Here's how the part is built. I have some questions about the finished solid (model axes, mm). A direction names the side the tool comes from. Coordinates: 2 decimals unless noted, no trailing zeros. Write each loop counter-clockwise with the first axis right and the second up, starting at its lowest first coordinate (ties: lowest second). Pieces come first, ordered by that corner, then holes. Notation, with made-up numbers: (18, -39.5) -> (41, -39.5) arc R27 ccw to (41, -15.5) -> close; hole circle Ø4 at (52, 20.25). An arc over 180 degrees is marked (long way). Answer in a Markdown table with one row per item. Add a question column.
from build123d import *

# Parameters (mm, degrees)
BOSS_EXTRUDE1_DEPTH = 15
SKETCH2_R           = 2.5
BOSS_EXTRUDE2_DEPTH = 2.5
FILLET1_R           = 1


with BuildPart() as part:
    # Sketch1 → Boss-Extrude1 (new, symmetric)
    with BuildSketch(Plane.XY):
        Polygon((-283.115153194, -200), (-283.115153194, 184.822832525), (-312.771891152, 214.573189293), (-282.723872007, 185), (282.728718813, 185), (312.776737958, 214.573189293), (283.12, 184.822832525), (283.12, -200), (313.12, -200), (313.12, 215), (-313.115153194, 215), (-313.115153194, -200), align=None)
    extrude(amount=BOSS_EXTRUDE1_DEPTH, both=True)

    # Sketch2 → Boss-Extrude2 (add, symmetric)
    with BuildSketch(Plane.ZY.offset(-283.12)):
        with BuildLine():
            Line((-15, -95.731232334), (-142.725217813, -153.297064452))
            ThreePointArc((-142.725217813, -153.297064452), (-144.870286213, -155.141843308), (-145.67073896, -157.855476088))
            Line((-145.67073896, -157.855476088), (-145.67073896, -195))
            ThreePointArc((-145.67073896, -195), (-144.206272866, -198.535533906), (-140.67073896, -200))
            Line((-140.67073896, -200), (140.67073896, -200))
            ThreePointArc((140.67073896, -200), (144.206272866, -198.535533906), (145.67073896, -195))
            Line((145.67073896, -195), (145.67073896, -157.855476088))
            ThreePointArc((145.67073896, -157.855476088), (144.870286213, -155.141843308), (142.725217813, -153.297064452))
            Line((142.725217813, -153.297064452), (15, -95.731232334))
            Line((15, -95.731232334), (-15, -95.731232334))
        make_face()
        with Locations(Location((-131.096268678, -157.855476088, 0), (0, 0, 270))):
            Circle(SKETCH2_R, mode=Mode.SUBTRACT)
        with Locations(Location((-131.096268678, -191.557763375, 0), (0, 0, 270))):
            Circle(SKETCH2_R, mode=Mode.SUBTRACT)
        with Locations(Location((131.096268678, -191.557763375, 0), (0, 0, 90))):
            Circle(SKETCH2_R, mode=Mode.SUBTRACT)
        with Locations(Location((131.096268678, -157.855476088, 0), (0, 0, 90))):
            Circle(SKETCH2_R, mode=Mode.SUBTRACT)
    boss_extrude2 = extrude(amount=BOSS_EXTRUDE2_DEPTH, both=True)

    # Mirror2: Boss-Extrude2 across plane
    add(boss_extrude2.mirror(Plane(origin=(0, 0, 0), x_dir=(0, 0, 1), z_dir=(1, 0, 0))))

    # Fillet1
    # the kernel refuses this fillet: 1 mm, written as the material it takes off along each edge
    with BuildSketch(Plane(origin=(-312.115153194, 214, -14), x_dir=(0, 0, -1), z_dir=(-1, 0, 0))) as fillet1_piece_1_section:
        Polygon((0, 0), (FILLET1_R * 1.02, 0), (FILLET1_R * 1.02, -FILLET1_R * 1.02), (0, -FILLET1_R * 1.02), align=None)
    fillet1_piece_1 = extrude(amount=FILLET1_R * 1.02, mode=Mode.PRIVATE)
    fillet1_piece_1 = fillet1_piece_1 - Plane(origin=(-312.115153194, 214, -14), x_dir=(0, -0.7071067811865475, 0.7071067811865475), z_dir=(-1, 0, 0)) * Sphere(FILLET1_R, mode=Mode.PRIVATE)
    add(fillet1_piece_1, mode=Mode.SUBTRACT)
    with BuildSketch(Plane(origin=(312.12, 214, -14), x_dir=(1, 0, 0), z_dir=(0, 1, 0))) as fillet1_piece_2_section:
        Polygon((0, 0), (FILLET1_R * 1.02, 0), (FILLET1_R * 1.02, FILLET1_R * 1.02), (0, FILLET1_R * 1.02), align=None)
    fillet1_piece_2 = extrude(amount=FILLET1_R * 1.02, mode=Mode.PRIVATE)
    fillet1_piece_2 = fillet1_piece_2 - Plane(origin=(312.12, 214, -14), x_dir=(-0.7071067811865475, 0, 0.7071067811865475), z_dir=(0, 1, 0)) * Sphere(FILLET1_R, mode=Mode.PRIVATE)
    add(fillet1_piece_2, mode=Mode.SUBTRACT)
    with BuildSketch(Plane(origin=(-312.115153194, 214, 14), x_dir=(0, 0, 1), z_dir=(-1, 0, 0))) as fillet1_piece_3_section:
        Polygon((0, 0), (FILLET1_R * 1.02, 0), (FILLET1_R * 1.02, FILLET1_R * 1.02), (0, FILLET1_R * 1.02), align=None)
    fillet1_piece_3 = extrude(amount=FILLET1_R * 1.02, mode=Mode.PRIVATE)
    fillet1_piece_3 = fillet1_piece_3 - Plane(origin=(-312.115153194, 214, 14), x_dir=(0, -0.7071067811865475, -0.7071067811865475), z_dir=(-1, 0, 0)) * Sphere(FILLET1_R, mode=Mode.PRIVATE)
    add(fillet1_piece_3, mode=Mode.SUBTRACT)
    with BuildSketch(Plane(origin=(312.12, 214, 14), x_dir=(1, 0, 0), z_dir=(0, 1, 0))) as fillet1_piece_4_section:
        Polygon((0, 0), (FILLET1_R * 1.02, 0), (FILLET1_R * 1.02, -FILLET1_R * 1.02), (0, -FILLET1_R * 1.02), align=None)
    fillet1_piece_4 = extrude(amount=FILLET1_R * 1.02, mode=Mode.PRIVATE)
    fillet1_piece_4 = fillet1_piece_4 - Plane(origin=(312.12, 214, 14), x_dir=(-0.7071067811865475, 0, -0.7071067811865475), z_dir=(0, 1, 0)) * Sphere(FILLET1_R, mode=Mode.PRIVATE)
    add(fillet1_piece_4, mode=Mode.SUBTRACT)
    with BuildSketch(Plane(origin=(-313.115153194, 214, -15), x_dir=(0, 0, 1), z_dir=(0, -1, 0)), Plane(origin=(313.12, -202.5, 15), x_dir=(-1, 0, 0), z_dir=(0, 1, 0))) as fillet1_piece_5:
        with BuildLine():
            CenterArc((FILLET1_R, -FILLET1_R), FILLET1_R, 90, 90)
            Line((0, -FILLET1_R), (0, 0))
            Line((0, 0), (FILLET1_R, 0))
        make_face()
    extrude(amount=416.5, mode=Mode.SUBTRACT)
    with BuildSketch(Plane(origin=(312.12, 215, -15), x_dir=(0, -1, 0), z_dir=(-1, 0, 0))) as fillet1_piece_6:
        with BuildLine():
            CenterArc((FILLET1_R, FILLET1_R), FILLET1_R, 180, 90)
            Line((0, FILLET1_R), (0, 0))
            Line((0, 0), (FILLET1_R, 0))
        make_face()
    extrude(amount=624.235153194, mode=Mode.SUBTRACT)
    with BuildSketch(Plane(origin=(313.12, -202.5, -15), x_dir=(-1, 0, 0), z_dir=(0, 1, 0)), Plane(origin=(-313.115153194, 214, 15), x_dir=(0, 0, -1), z_dir=(0, -1, 0))) as fillet1_piece_7:
        with BuildLine():
            CenterArc((FILLET1_R, FILLET1_R), FILLET1_R, 180, 90)
            Line((0, FILLET1_R), (0, 0))
            Line((0, 0), (FILLET1_R, 0))
        make_face()
    extrude(amount=416.5, mode=Mode.SUBTRACT)
    with BuildSketch(Plane(origin=(283.12, 187.322832525, -15), x_dir=(1, 0, 0), z_dir=(0, -1, 0))) as fillet1_piece_8_section:
        with BuildLine():
            CenterArc((FILLET1_R, FILLET1_R), FILLET1_R, 180, 90)
            Line((0, FILLET1_R), (0, 0))
            Line((0, 0), (FILLET1_R, 0))
        make_face()
    fillet1_piece_8 = extrude(amount=283.054064858, mode=Mode.PRIVATE)
    fillet1_piece_8 = split(fillet1_piece_8, bisect_by=Plane(origin=(212.904028108, 116.278704743, -14.776762441), z_dir=(0.7014530599300108, -0.712715654882664, 0)), keep=Keep.TOP, mode=Mode.PRIVATE)
    add(fillet1_piece_8, mode=Mode.SUBTRACT)
    with BuildSketch(Plane(origin=(-285.223872007, 185, -15), x_dir=(0, 1, 0), z_dir=(1, 0, 0))) as fillet1_piece_9_section:
        with BuildLine():
            CenterArc((FILLET1_R, FILLET1_R), FILLET1_R, 180, 90)
            Line((0, FILLET1_R), (0, 0))
            Line((0, 0), (FILLET1_R, 0))
        make_face()
    fillet1_piece_9 = extrude(amount=570.45259082, mode=Mode.PRIVATE)
    fillet1_piece_9 = split(fillet1_piece_9, bisect_by=Plane(origin=(139.225783569, 43.764750927, -14.776706333), z_dir=(-0.7014530599300108, 0.712715654882664, 0)), keep=Keep.TOP, mode=Mode.PRIVATE)
    fillet1_piece_9 = split(fillet1_piece_9, bisect_by=Plane(origin=(-142.20285466, 43.465709552, -14.776706333), z_dir=(0.7082202214843082, 0.7059915848512059, 0)), keep=Keep.TOP, mode=Mode.PRIVATE)
    add(fillet1_piece_9, mode=Mode.SUBTRACT)
    with BuildSketch(Plane(origin=(-313.115153194, -200, 17.5), x_dir=(1, 0, 0), z_dir=(0, 0, -1))) as fillet1_piece_10:
        with BuildLine():
            CenterArc((FILLET1_R, -FILLET1_R), FILLET1_R, 90, 90)
            Line((0, -FILLET1_R), (0, 0))
            Line((0, 0), (FILLET1_R, 0))
        make_face()
    extrude(amount=35, mode=Mode.SUBTRACT)
    with BuildSketch(Plane(origin=(-313.115153194, 215, 14), x_dir=(0, -1, 0), z_dir=(0, 0, -1))) as fillet1_piece_11:
        with BuildLine():
            CenterArc((FILLET1_R, -FILLET1_R), FILLET1_R, 90, 90)
            Line((0, -FILLET1_R), (0, 0))
            Line((0, 0), (FILLET1_R, 0))
        make_face()
    extrude(amount=28, mode=Mode.SUBTRACT)
    with BuildSketch(Plane(origin=(313.12, 215, -14), x_dir=(-1, 0, 0), z_dir=(0, 0, 1))) as fillet1_piece_12:
        with BuildLine():
            CenterArc((FILLET1_R, FILLET1_R), FILLET1_R, 180, 90)
            Line((0, FILLET1_R), (0, 0))
            Line((0, 0), (FILLET1_R, 0))
        make_face()
    extrude(amount=28, mode=Mode.SUBTRACT)
    with BuildSketch(Plane(origin=(-285.223872007, 185, 15), x_dir=(0, 1, 0), z_dir=(1, 0, 0))) as fillet1_piece_13_section:
        with BuildLine():
            CenterArc((FILLET1_R, -FILLET1_R), FILLET1_R, 90, 90)
            Line((0, -FILLET1_R), (0, 0))
            Line((0, 0), (FILLET1_R, 0))
        make_face()
    fillet1_piece_13 = extrude(amount=570.45259082, mode=Mode.PRIVATE)
    fillet1_piece_13 = split(fillet1_piece_13, bisect_by=Plane(origin=(139.225783569, 43.764750927, 14.776706333), z_dir=(-0.7014530599300108, 0.712715654882664, 0)), keep=Keep.TOP, mode=Mode.PRIVATE)
    fillet1_piece_13 = split(fillet1_piece_13, bisect_by=Plane(origin=(-142.20285466, 43.465709552, 14.776706333), z_dir=(0.7082202214843082, 0.7059915848512059, 0)), keep=Keep.TOP, mode=Mode.PRIVATE)
    add(fillet1_piece_13, mode=Mode.SUBTRACT)
    with BuildSketch(Plane(origin=(313.12, -200, -17.5), x_dir=(0, 1, 0), z_dir=(0, 0, 1))) as fillet1_piece_14:
        with BuildLine():
            CenterArc((FILLET1_R, FILLET1_R), FILLET1_R, 180, 90)
            Line((0, FILLET1_R), (0, 0))
            Line((0, 0), (FILLET1_R, 0))
        make_face()
    extrude(amount=35, mode=Mode.SUBTRACT)
    with BuildSketch(Plane(origin=(282.728718813, 185, -16.023890127), x_dir=(0.7127156548826233, 0.701453059930052, 0), z_dir=(0, 0, 1)), Plane(origin=(-282.723872007, 185, -16.023890127), x_dir=(1, 0, 0), z_dir=(0, 0, 1))) as fillet1_piece_15:
        with BuildLine():
            CenterArc((FILLET1_R * 0.409556050901, FILLET1_R), FILLET1_R, 225.456300233, 44.543699767)
            Line((-FILLET1_R * 0.291897009029, FILLET1_R * 0.287284345117), (0, 0))
            Line((0, 0), (FILLET1_R * 0.409556050901, 0))
        make_face()
    extrude(amount=32.047780255, mode=Mode.SUBTRACT)
    with BuildSketch(Plane(origin=(283.12, 187.322832525, 15), x_dir=(1, 0, 0), z_dir=(0, -1, 0))) as fillet1_piece_16_section:
        with BuildLine():
            CenterArc((FILLET1_R, -FILLET1_R), FILLET1_R, 90, 90)
            Line((0, -FILLET1_R), (0, 0))
            Line((0, 0), (FILLET1_R, 0))
        make_face()
    fillet1_piece_16 = extrude(amount=283.054064858, mode=Mode.PRIVATE)
    fillet1_piece_16 = split(fillet1_piece_16, bisect_by=Plane(origin=(212.904028108, 116.278704743, 14.776762441), z_dir=(0.7014530599300108, -0.712715654882664, 0)), keep=Keep.TOP, mode=Mode.PRIVATE)
    add(fillet1_piece_16, mode=Mode.SUBTRACT)
    with BuildSketch(Plane(origin=(312.12, 215, 15), x_dir=(0, -1, 0), z_dir=(-1, 0, 0))) as fillet1_piece_17:
        with BuildLine():
            CenterArc((FILLET1_R, -FILLET1_R), FILLET1_R, 90, 90)
            Line((0, -FILLET1_R), (0, 0))
            Line((0, 0), (FILLET1_R, 0))
        make_face()
    extrude(amount=624.235153194, mode=Mode.SUBTRACT)
    with BuildSketch(Plane(origin=(-283.115153194, -95.731232334, -15), x_dir=(-1, 0, 0), z_dir=(0, 1, 0))) as fillet1_piece_18_section:
        with BuildLine():
            CenterArc((FILLET1_R, FILLET1_R), FILLET1_R, 180, 90)
            Line((0, FILLET1_R), (0, 0))
            Line((0, 0), (FILLET1_R, 0))
        make_face()
    fillet1_piece_18 = extrude(amount=283.054064858, mode=Mode.PRIVATE)
    fillet1_piece_18 = split(fillet1_piece_18, bisect_by=Plane(origin=(-142.946899789, 44.212103442, -14.61922956), z_dir=(-0.7082202214843082, -0.7059915848512059, 0)), keep=Keep.TOP, mode=Mode.PRIVATE)
    add(fillet1_piece_18, mode=Mode.SUBTRACT)
    with BuildSketch(Plane(origin=(-283.115153194, -95.731232334, 15), x_dir=(-1, 0, 0), z_dir=(0, 1, 0))) as fillet1_piece_19_section:
        with BuildLine():
            CenterArc((FILLET1_R, -FILLET1_R), FILLET1_R, 90, 90)
            Line((0, -FILLET1_R), (0, 0))
            Line((0, 0), (FILLET1_R, 0))
        make_face()
    fillet1_piece_19 = extrude(amount=283.054064858, mode=Mode.PRIVATE)
    fillet1_piece_19 = split(fillet1_piece_19, bisect_by=Plane(origin=(-142.946899789, 44.212103442, 14.61922956), z_dir=(-0.7082202214843082, -0.7059915848512059, 0)), keep=Keep.TOP, mode=Mode.PRIVATE)
    add(fillet1_piece_19, mode=Mode.SUBTRACT)


solid = part.part
Q1. Imagine slicing it at C-C on x = -172.5. Please give me the cut outline in (y, z).
Q2. Imagine slicing it at D-D on y = -145.5. Please give me the cut outline in (x, z).
Q3. Imagine slicing it at B-B on z = 71.5. Please give me the cut outline in (x, y).
Q4. If we mould it in two halves opening along Z, with no side actions, what happens to faces 1 (the flat face through (-4, 185, 0)), 2 (the flat face through (-4, 200, 15)), 3 (the flat face through (298.16, 199.91, 0.21))? For each: pulls with the +Z half, pulls with the -Z half, needs draft (parallel to the pull), parting line crosses it, or undercut.
Q5. I'm going to push flat-ended pins straight in: P1, Ø4, axis at y = -157.86, z = -131.1, coming from the -X side; P2, Ø14, axis at x = -3, z = -2, coming from the -Y side; P3, Ø22.5, axis at x = -296.5, y = -30, coming from the -Z side; P4, Ø6, axis at y = -191.56, z = -131.1, coming from the +X side. Where does each tip first touch, or does it pass through?
Q6. For faces 4 (the flat face through (285.62, -159, -67)), 5 (the flat face through (280.62, -159, -2)), 6 (the flat face through (-298.102, 200.135, 0.21)), 7 (the flat face through (283.12, 47, 0)), which set-ups out of +Z, -Z, +X, -X, +Y, -Y let a thin tool reach every point of the face, with its end or its side?
Q7. Imagine slicing it at A-A on y = 94. Please give me the cut outline in (x, z), plus the area to 3 significant figures.
Q8. I need wall thicknesses on line 1 (X direction, y = -169, z = 92); line 2 (X direction, y = -90, z = 9); line 3 (Z direction, x = -120.5, y = 188). Which ranges of each line are inside material? Lowest first, please. Write a range as [from, to].
Result sheet:
| question | item | result |
|---|---|---|
| 1 | outline | (185, -14) arc R1 ccw to (186, -15) -> (214, -15) arc R1 ccw to (215, -14) -> (215, 14) arc R1 ccw to (214, 15) -> (186, 15) arc R1 ccw to (185, 14) -> close |
| 2 | outline | (-313.12, -14) arc R1 ccw to (-312.12, -15) -> (-285.62, -15) -> (-285.62, -125.43) -> (-280.62, -125.43) -> (-280.62, 125.43) -> (-285.62, 125.43) -> (-285.62, 15) -> (-312.12, 15) arc R1 ccw to (-313.12, 14) -> close; (280.62, -125.43) -> (285.62, -125.43) -> (285.62, -15) -> (312.12, -15) arc R1 ccw to (313.12, -14) -> (313.12, 14) arc R1 ccw to (312.12, 15) -> (285.62, 15) -> (285.62, 125.43) -> (280.62, 125.43) -> close |
| 3 | outline | (-285.62, -200) -> (-280.62, -200) -> (-280.62, -121.2) -> (-285.62, -121.2) -> close; (280.62, -200) -> (285.62, -200) -> (285.62, -121.2) -> (280.62, -121.2) -> close |
| 4 | face 1 | needs draft |
| 4 | face 2 | pulls with the +Z half |
| 4 | face 3 | undercut |
| 5 | P1 | passes through |
| 5 | P2 | stops at y = 185 |
| 5 | P3 | stops at z = -15 |
| 5 | P4 | stops at x = 285.62 |
| 6 | face 4 | -Z, +X, +Y, -Y |
| 6 | face 5 | +Z, -Z, -Y |
| 6 | face 6 | none |
| 6 | face 7 | +Z, -Z |
| 7 | outline | (-313.12, -14) arc R1 ccw to (-312.12, -15) -> (-284.12, -15) arc R1 ccw to (-283.12, -14) -> (-283.12, 14) arc R1 ccw to (-284.12, 15) -> (-312.12, 15) arc R1 ccw to (-313.12, 14) -> close; (283.12, -14) arc R1 ccw to (284.12, -15) -> (312.12, -15) arc R1 ccw to (313.12, -14) -> (313.12, 14) arc R1 ccw to (312.12, 15) -> (284.12, 15) arc R1 ccw to (283.12, 14) -> close |
| 7 | area | 1,800 mm^2 |
| 8 | line 1 | x = [-285.62, -280.62], [280.62, 285.62] |
| 8 | line 2 | x = [-313.12, -283.12], [283.12, 313.12] |
| 8 | line 3 | z = [-15, 15] |
